Autodesk Inventor part; units mm, degrees
ref_plane "YZ Plane" through (0, 0, 0) normal (1, 0, 0) x (0, 1, 0)
ref_plane "XZ Plane" through (0, 0, 0) normal (0, 1, 0) x (-1, 0, 0)
ref_plane "XY Plane" through (0, 0, 0) normal (0, 0, 1) x (1, 0, 0)
sketch "Sketch1" plane through (0, 0, 0) normal (0, 1, 0) x (-1, 0, 0)
  line L0 (0, 0) -> (50.8, 0)
  line L1 (50.8, 0) -> (50.8, -3.175)
  line L2 (50.8, -3.175) -> (0, -3.175)
  line L3 (0, -3.175) -> (0, 0)
  line L4 (0, 0) -> (3.175, 0)
  line L5 (3.175, 0) -> (3.175, -50.8)
  line L6 (3.175, -50.8) -> (0, -50.8)
  line L7 (0, -50.8) -> (0, 0)
  dimension "d0" = 50.8
  dimension "d1" = 3.175
  dimension "d2" = 3.175
  dimension "d3" = 50.8
extrude "Extrusion1" add sketch "Sketch1" along normal blind 50.8
sketch "Sketch2" plane through (-50.8, 0, 0) normal (0, 0, 1) x (1, 0, 0)
  line L0 (0, 50.8) -> (25.4, 50.8)
  line L1 (25.4, 50.8) -> (25.4, 0)
  line L2 (25.4, 0) -> (0, 0)
  line L3 (0, 0) -> (0, 50.8)
  point P0 (50.8, 0)
  dimension "d6" = 25.4
  dimension "d7" = 50.8
extrude "Extrusion2" cut sketch "Sketch2" against normal blind 50.8
sketch "Sketch3" plane through (0, 0, 0) normal (1, 0, 0) x (0, 0, -1)
  line L0 (0, 50.8) -> (50.8, 50.8)
  line L1 (0, 0) -> (0, 50.8)
  line L2 (0, 0) -> (50.8, 0)
  line L3 (50.8, 0) -> (50.8, 50.8)
  line L4 (3.175, 0) -> (3.175, 50.8)
  line L5 (0, 0) -> (3.175, 0)
  line L6 (0, 50.8) -> (0, 0)
  line L7 (3.175, 50.8) -> (0, 50.8)
  circle A0 centre (12.7, 38.1) radius 3.175 construction
  line L8 (3.175, 50.8) -> (9.8303, 36.7415) construction
  line L9 (0, 50.8) -> (50.8, 50.8) construction
  line L10 (22.225, 50.8) -> (15.5697, 36.7415) construction
  line L11 (3.175, 50.8) -> (9.8303, 36.7415)
  line L12 (22.225, 50.8) -> (15.5697, 36.7415)
  arc A1 (9.8303, 36.7415) -> (15.5697, 36.7415) centre (12.7, 38.1) ccw
  line L13 (3.175, 50.8) -> (22.225, 50.8)
  dimension "d10" = 6.35
  dimension "d11" = 19.05
  dimension "d12" = 9.525
  dimension "d13" = 12.7
extrude "Extrusion3" cut sketch "Sketch3" against normal blind 50.8 contours L0 L12 A1 L11
sketch "Sketch4" plane through (0, 0, 0) normal (1, 0, 0) x (0, 0, -1)
  line L0 (50.8, 50.8) -> (38.1, 50.8)
  line L1 (22.225, 50.8) -> (50.8, 50.8)
  line L2 (50.8, 50.8) -> (50.8, 25.4)
  line L3 (50.8, 0) -> (50.8, 50.8)
  line L4 (50.8, 25.4) -> (38.1, 50.8)
  point P0 (0, 0)
  dimension "d16" = 12.7
  dimension "d17" = 25.4
extrude "Extrusion4" cut sketch "Sketch4" against normal blind 50.8
sketch "Sketch5" plane through (0, 0, 0) normal (1, 0, 0) x (0, 0, -1)
  line L0 (0, 0) -> (0, 50.8)
  line L1 (0, 0) -> (50.8, 0)
  line L2 (50.8, 0) -> (50.8, 25.4)
  point P0 (15.875, 12.7)
  point P1 (41.275, 12.7)
  dimension "d20" = 15.875
  dimension "d21" = 12.7
  dimension "d22" = 12.7
  dimension "d23" = 9.525
hole "Hole1" at (0, 12.7, -15.875) at (0, 12.7, -41.275) direction (-1, 0, 0) diameter 6.35 end through all
properties part number "front tab 2x2" material "Aluminum 6061"
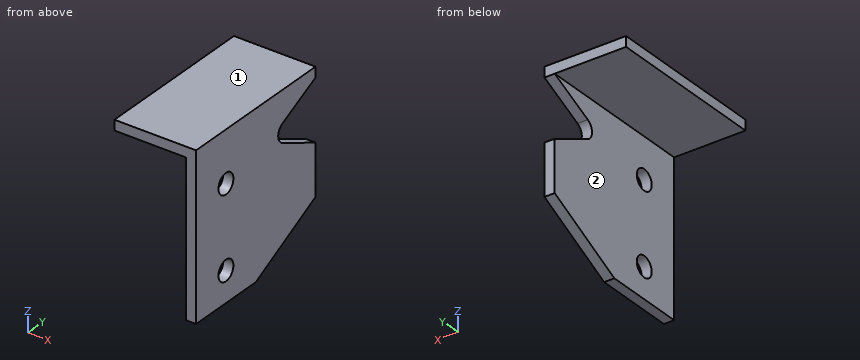
Model file for the job. Use its own axes, mm. Face numbers are marked on the shaded views. A direction names the side the tool comes from. Round coordinates to 2 decimals unless told otherwise and drop trailing zeros. Loops run counter-clockwise (first coordinate to the right, second up) from the corner with the lowest first, then second, coordinate; pieces in that order, holes last.
1. Band-saw the part on C-C, the plane z = -40. List the corners of the cut face in (x, y) (3 decimals), and give its area (3 significant figures).
Check values:
outline: (-3.175, 0) - (0, 0) - (0, 9.792) - (-3.175, 9.792) - close; (-3.175, 15.608) - (0, 15.608) - (0, 47) - (-3.175, 47) - close
area: 131 mm2
2. Wall check: probe 1 along Z at (x, y) = (-1.65, 12.7); probe 2 along X at (y, z) = (31, -28) (3 decimals). Give the ranges that are in metal, low to high.
Check values:
probe 1: z = -50.8 to -44.45, -38.1 to -19.05, -12.7 to 0
probe 2: x = -3.175 to 0
3. Band-saw the part on B-B, the plane y = 22. List the corners of the cut face in (x, z) (3 decimals), and give its area (3 significant figures).
Check values:
outline: (-25.4, -3.175) - (-3.175, -3.175) - (-3.175, -50.8) - (0, -50.8) - (0, 0) - (-25.4, 0) - close
area: 232 mm2
4. Band-saw the part on D-D, the plane x = -11.5. List the corners of the cut face in (y, z) (3 decimals), and give its area (3 significant figures).
Check values:
outline: (0, -3.175) - (50.8, -3.175) - (50.8, 0) - (0, 0) - close
area: 161 mm2
5. Tool access for the marked faces 1 and 2: list every direction of +Z, -Z, +X, -X, +Y, -Y with a clear straight run to the whole face (end or side of a thin tool).
Check values:
face 1: +Z, +X, -X, +Y, -Y
face 2: -Z, -X, +Y, -Y
6. Band-saw the part on A-A, the plane y = 12.7. List the corners of the cut face in (x, z) (3 decimals), and give its area (3 significant figures).
Check values:
outline: (-25.4, -3.175) - (-3.175, -3.175) - (-3.175, -12.7) - (0, -12.7) - (0, 0) - (-25.4, 0) - close; (-3.175, -50.8) - (0, -50.8) - (0, -44.45) - (-3.175, -44.45) - close; (-3.175, -38.1) - (0, -38.1) - (0, -19.05) - (-3.175, -19.05) - close
area: 192 mm2
7. Drop flat-ended pins along their axis: P1, Ø5, axis at y = 21, z = -11.5, coming from the -X side (3 decimals); P2, Ø6.5, axis at x = -19, y = 22, coming from the -Z side (3 decimals); P3, Ø5.5, axis at y = 12.7, z = -15.875, coming from the +X side. Give the stop position or say it passes through.
Check values:
P1: stops at x = -3.175
P2: stops at z = -3.175
P3: passes through
